Job drawing, mm, ordinate dimensions from the low corner. One solid piece. A direction names the side the tool comes from. Round coordinates to 2 decimals unless told otherwise and drop trailing zeros. Loops run counter-clockwise (first coordinate to the right, second up) from the corner with the lowest first, then second, coordinate; pieces in that order, holes last. Notation, with made-up numbers: (86, -13.5) - (120, -13.5) arc R17 ccw to (120, -9.5) - close; hole circle Ø8 at (7.25, 69.25). An arc over 180 degrees is marked (long way). Answer as CSV lines item,"result". Start each with the question number.
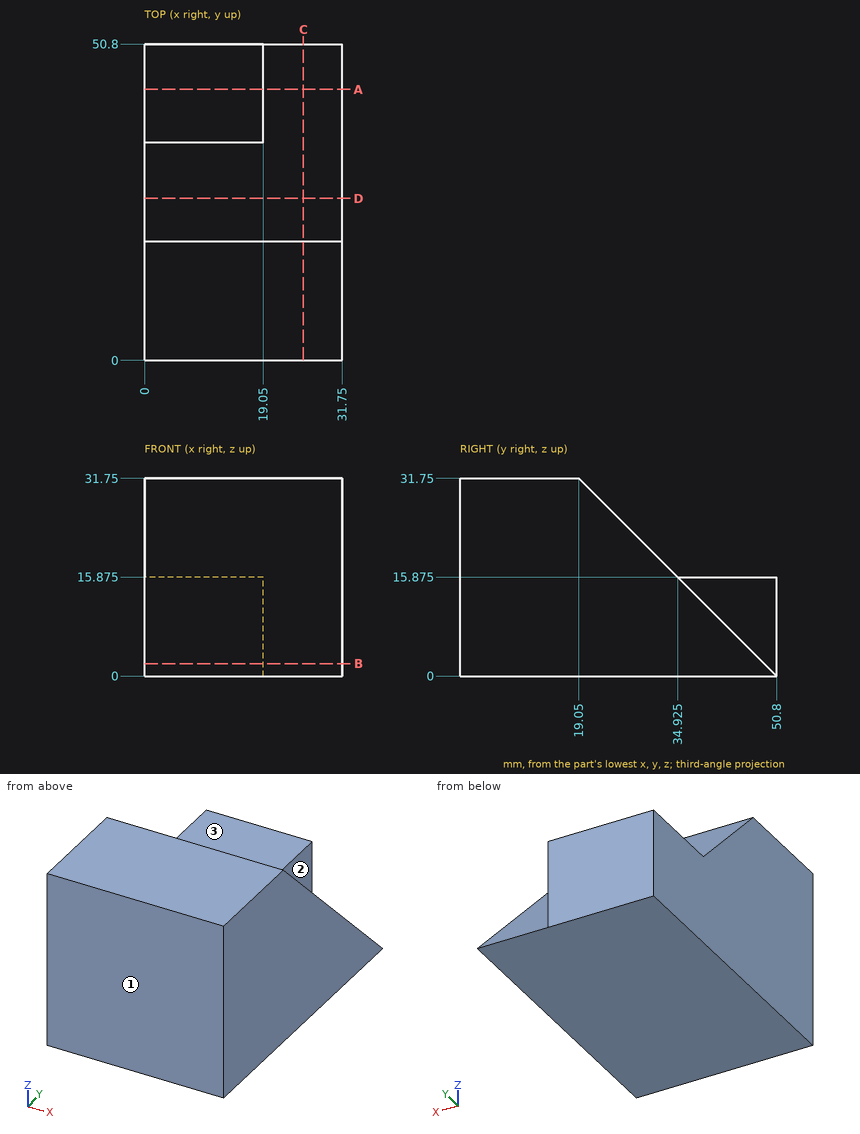
Q1. Pin check, flat tip, straight feed: pin 1 Ø8 at (x, y) = (11.5, 39) entering from +Z (3 decimals). Stop position of the tip, or through.
Q2. Band-saw the part on A-A, the plane y = 43.5. List the corners of the cut face in (x, z) (3 decimals), then the cut area to 3 significant figures.
Q3. Tool access for the marked faces 1, 2 and 3: list every direction of +Z, -Z, +X, -X, +Y, -Y with a clear straight run to the whole face (end or side of a thin tool).
Q4. Band-saw the part on D-D, the plane y = 26. List the corners of the cut face in (x, z), then the cut area to 3 significant figures.
Q5. Band-saw the part on B-B, the plane z = 2. List the corners of the cut face in (x, y).
Q6. Band-saw the part on C-C, the plane x = 25.5. List the corners of the cut face in (y, z).
Q7. Wall check: probe 1 along X at (y, z) = (47.5, 13); probe 2 along Z at (x, y) = (16, 47) (3 decimals); probe 3 along Z at (x, y) = (9.5, 29.5). Give the ranges that are in metal, low to high. Write a range as [from, to].
Reported:
1,pin 1,"stops at z = 15.875"
2,outline,"(0, 0) - (31.75, 0) - (31.75, 7.3) - (19.05, 7.3) - (19.05, 15.875) - (0, 15.875) - close"
2,area,"395 mm2"
3,face 1,"+Z, -Z, +X, -X, -Y"
3,face 2,"+Z, +X, +Y"
3,face 3,"+Z, +X, -X, +Y"
4,outline,"(0, 0) - (31.75, 0) - (31.75, 24.8) - (0, 24.8) - close"
4,area,"787 mm2"
5,outline,"(0, 0) - (31.75, 0) - (31.75, 48.8) - (19.05, 48.8) - (19.05, 50.8) - (0, 50.8) - close"
6,outline,"(0, 0) - (50.8, 0) - (19.05, 31.75) - (0, 31.75) - close"
7,probe 1,"x = [0, 19.05]"
7,probe 2,"z = [0, 15.875]"
7,probe 3,"z = [0, 21.3]"
